Autodesk Inventor part; units mm, degrees
ref_plane "YZ Plane" through (0, 0, 0) normal (1, 0, 0) x (0, 1, 0)
ref_plane "XZ Plane" through (0, 0, 0) normal (0, 1, 0) x (-1, 0, 0)
ref_plane "XY Plane" through (0, 0, 0) normal (0, 0, 1) x (1, 0, 0)
sketch "Sketch1" plane through (0, 0, 0) normal (1, 0, 0) x (0, 1, 0)
  line L0 (0.2223, 0) -> (56.1023, 0)
  line L1 (56.1023, 0) -> (56.1023, -44.45)
  line L2 (56.1023, -44.45) -> (-7.3977, -44.45)
  line L3 (-7.3977, -44.45) -> (-7.3977, -42.8625)
  line L4 (-7.3977, -42.8625) -> (-10.5727, -42.8625)
  line L5 (-10.5727, -42.8625) -> (-10.5727, -41.275)
  line L6 (-10.5727, -41.275) -> (52.9273, -41.275)
  line L7 (52.9273, -41.275) -> (52.9273, -3.175)
  line L8 (52.9273, -3.175) -> (0.2223, -3.175)
  line L9 (0.2223, -3.175) -> (0.2223, 0)
  line L10 (68.5874, 139.7) -> (-16.5119, 139.7)
  point P0 (0, 0)
  dimension "d0" = 55.88
  dimension "d1" = 44.45
  dimension "d2" = 63.5
  dimension "d3" = 1.5875
  dimension "d4" = 90
  dimension "d5" = 3.175
  dimension "d6" = 1.5875
  dimension "d7" = 63.5
  dimension "d8" = 38.1
  dimension "d9" = 90
  dimension "d10" = 139.7
revolve "Revolution1" add sketch "Sketch1" angle 240 about axis through (0, 68.5874, 139.7) along (0, -1, 0)
fillet "Fillet1" radius 6.35 1 edges at (159.4786, 56.1023, 231.775)
fillet "Fillet2" radius 6.35 1 edges at (120.9837, 56.1023, 209.55)
properties part number "Top"
Input: part model. Units: mm. Frame: model coordinates. A direction names the side the tool comes from. Give positions to 0.01 mm unless a question says otherwise; leave off trailing zeros.
1. Draft query along Z for faces 1 (the face through (-157.25, 32.49, 230.49)), 2 (the face through (0, 32, -42)), 3 (the face through (119, 0.222, 214)). Return one class per face: released by +Z, released by -Z, zero draft, split by the parting line, or undercut.
Computed:
face 1: released by -Z
face 2: zero draft
face 3: undercut
2. Line query: probe 1 along X at (y, z) = (21, 139); probe 2 along Z at (x, y) = (31, 17.5); probe 3 along Z at (x, y) = (44.5, 5). Output: solid intervals per line, ascending.
Computed:
probe 1: x = 139.7 to 142.87, 180.97 to 184.15
probe 2: z = -41.82 to -38.6, 0.23 to 3.48, 275.92 to 279.17, 318 to 321.22
probe 3: z = -38.99 to -35.72, 3.93 to 7.28, 272.12 to 275.47, 315.12 to 318.39
3. Pin query (flat end, axial travel): pin 1 Ø3 at (x, y) = (-111.5, 48.5) entering from -Z; pin 2 Ø12 at (x, y) = (51, 49) entering from +Z; pin 3 Ø22 at (y, z) = (25.5, -32.5) entering from -X. Return the tip coordinate at first contact, or that it passes through.
Computed:
pin 1: stops at z = 221.84
pin 2: stops at z = 318.27
pin 3: stops at x = 0
4. Set-up query: faces 4 (the face through (160.71, -9.01, 226.31)), 5 (the face through (123, 56.102, 220)). Return all of +Z, -Z, +X, -X, +Y, -Y with unobstructed straight access to the full face (end or side cutting, diameter ignored); none if empty.
Computed:
face 4: -Y
face 5: +Z, -Z, +X, -X, +Y
